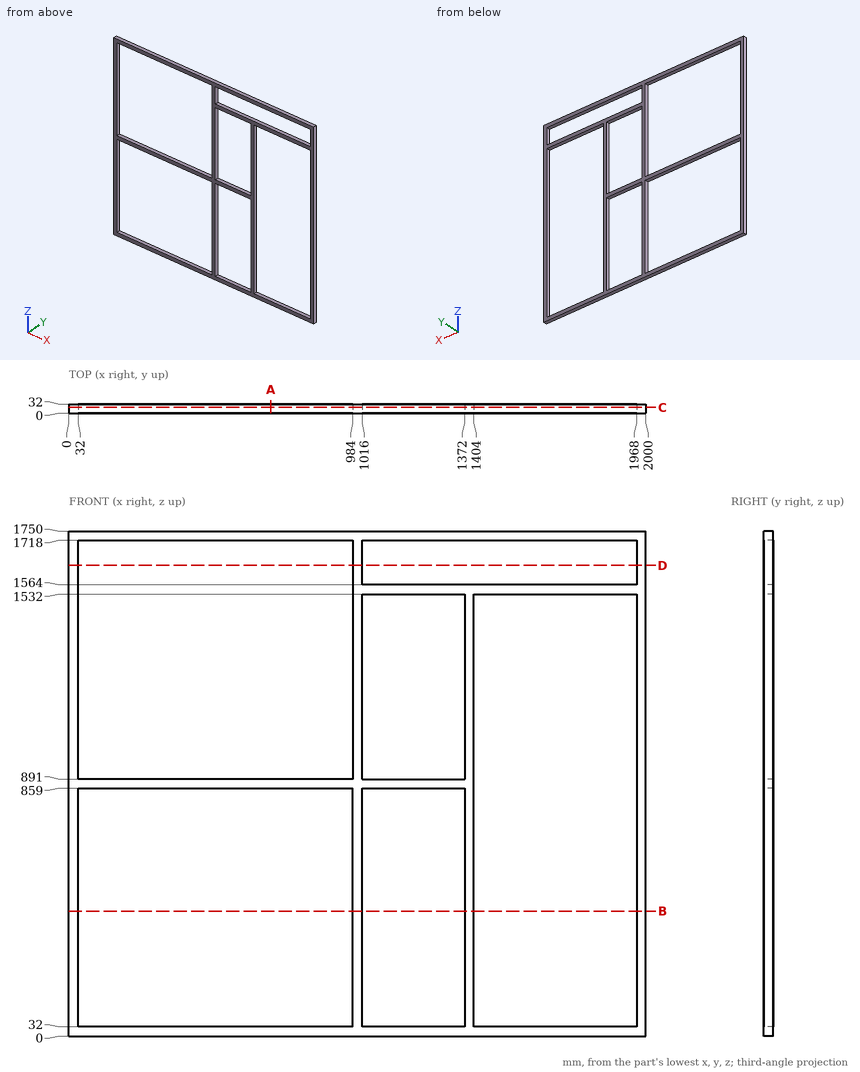
Input: dimensioned drawing with shaded views. Units: mm. Origin: part minimum x, y, z. Round coordinates to 2 decimals unless told otherwise and drop trailing zeros. Loops run counter-clockwise (first coordinate to the right, second up) from the corner with the lowest first, then second, coordinate; pieces in that order, holes last. Notation, with made-up numbers: (36.5, -8) -> (51.5, -8) arc R22 cw to (51.5, 12) -> close; hole circle Ø10 at (-23.5, -30). An arc over 180 degrees is marked (long way). Answer as a JSON object with one key per item and string values. Group by question number.
Q1. Section query C-C (y = 20). Output: boundary loops of the cut face in (x, z), plus the area to 3 significant figures.
Q2. Section query A-A (x = 700). Output: boundary loops of the cut face in (y, z).
Q3. Ray query, line 1 (Z direction, x = 365, y = 17); line 2 (X direction, y = 23.5, z = 169); line 3 (Z direction, x = 1822.5, y = 21). Return the intervals inside material, ascending. Write a range as from..to.
Q4. Section query D-D (z = 1631.5). Output: boundary loops of the cut face in (x, y), plus the area to 3 significant figures.
Q5. Section query B-B (z = 433). Output: boundary loops of the cut face in (x, y).
Completed:
{
 "1": {"outline": "(0, 0) -> (2000, 0) -> (2000, 1750) -> (0, 1750) -> close; hole (32, 32) -> (984, 32) -> (984, 859) -> (32, 859) -> close; hole (32, 891) -> (984, 891) -> (984, 1718) -> (32, 1718) -> close; hole (1016, 32) -> (1372, 32) -> (1372, 859) -> (1016, 859) -> close; hole (1016, 891) -> (1372, 891) -> (1372, 1532) -> (1016, 1532) -> close; hole (1016, 1564) -> (1968, 1564) -> (1968, 1718) -> (1016, 1718) -> close; hole (1404, 32) -> (1968, 32) -> (1968, 1532) -> (1404, 1532) -> close", "area": "410,000 mm²"},
 "2": {"outline": "(0, 0) -> (32, 0) -> (32, 32) -> (0, 32) -> close; (0, 859) -> (32, 859) -> (32, 891) -> (0, 891) -> close; (0, 1718) -> (32, 1718) -> (32, 1750) -> (0, 1750) -> close"},
 "3": {"line 1": "0..32, 859..891, 1718..1750", "line 2": "0..32, 984..1016, 1372..1404, 1968..2000", "line 3": "0..32, 1532..1564, 1718..1750"},
 "4": {"outline": "(0, 0) -> (32, 0) -> (32, 32) -> (0, 32) -> close; (984, 0) -> (1016, 0) -> (1016, 32) -> (984, 32) -> close; (1968, 0) -> (2000, 0) -> (2000, 32) -> (1968, 32) -> close", "area": "3,070 mm²"},
 "5": {"outline": "(0, 0) -> (32, 0) -> (32, 32) -> (0, 32) -> close; (984, 0) -> (1016, 0) -> (1016, 32) -> (984, 32) -> close; (1372, 0) -> (1404, 0) -> (1404, 32) -> (1372, 32) -> close; (1968, 0) -> (2000, 0) -> (2000, 32) -> (1968, 32) -> close"}
}
